```python
from build123d import *

# Parameters (mm, degrees)
SKETCH_2_R      = 3
EXTRUDE_1_DEPTH = 1.6


with BuildPart() as part:
    # 스케치2 → 보스-돌출1 (new body)
    with BuildSketch(Plane(origin=(0, 0, 0), x_dir=(0, 0, -1), z_dir=(1, 0, 0))):
        with BuildLine():
            Line((-13.45, 1.3), (-11.65, 1.3))
            Line((-11.65, 1.3), (-11.65, 0.5))
            Line((-11.65, 0.5), (-7.05, 0.5))
            Line((-7.05, 0.5), (-7.05, 1.3))
            Line((-7.05, 1.3), (-2, 1.3))
            Line((-2, 1.3), (-2, 2.063932023))
            ThreePointArc((-2, 2.063932023), (0, 7.3), (2, 2.063932023))
            Line((2, 2.063932023), (2, 1.3))
            Line((2, 1.3), (7.05, 1.3))
            Line((7.05, 1.3), (7.05, 0.5))
            Line((7.05, 0.5), (11.65, 0.5))
            Line((11.65, 0.5), (11.65, 1.3))
            Line((11.65, 1.3), (13.45, 1.3))
            Line((13.45, 1.3), (13.45, 10.3))
            Line((13.45, 10.3), (-11.45, 10.3))
            Line((-11.45, 10.3), (-11.45, 12.3))
            Line((-11.45, 12.3), (-13.45, 12.3))
            Line((-13.45, 12.3), (-13.45, 1.3))
        make_face()
        with Locations((-7.05, 6.25)):
            Circle(SKETCH_2_R, mode=Mode.SUBTRACT)
        with Locations((7.05, 6.25)):
            Circle(SKETCH_2_R, mode=Mode.SUBTRACT)
    extrude(amount=EXTRUDE_1_DEPTH)


solid = part.part
```
Geometry: final body of the model. Coordinates: model frame, mm. A direction names the side the tool comes from. Coordinates: 2 decimals unless noted, no trailing zeros. Order: outer loops, then holes, each group sorted by start corner. A loop starts at its lowest first (then second) coordinate and runs counter-clockwise, first axis right, second up. Notation, with made-up numbers: (-38, 30) - (15, 30) arc R37 ccw to (15, 66) - close; hole circle Ø4 at (38.25, 59). An arc over 180 degrees is marked (long way). Return JSON: item names as keys, results as strings. Group by question number.
1. Set-up query: faces 4 (the face through (1, 0.5, -9)), 5 (the face through (1, 1.3, -4)), 6 (the face through (1, 10.3, -1)), 7 (the face through (1, 1.3, -13)), 8 (the face through (1, 1.3, 13)). Return all of +Z, -Z, +X, -X, +Y, -Y with unobstructed straight access to the full face (end or side cutting, diameter ignored); none if empty.
2. Cut plane B-B (x = 0.85). Output: boundary loops of the cut face in (y, z).
3. Cut plane D-D (z = 9). Output: boundary loops of the cut face in (x, y), plus the area to 3 significant figures.
4. Material intervals for line 1 along Z through (x, y) = (0.6, 4); line 2 along Z through (x, y) = (0.25, 4.25); line 3 along Z through (x, y) = (0.45, 9), sorted ascending. Write a range as [from, to].
5. Pull-direction query (Z, two-part tool) for faces 1 (the face through (1, 1.3, 5)), 2 (the face through (1, 7, 13.45)), 3 (the face through (1, 11, 11.45)); classes: pulls with the +Z half, pulls with the -Z half, needs draft (parallel to the pull), parting line crosses it, or undercut.
6. Cut plane A-A (y = 2.5). Output: boundary loops of the cut face in (x, z), plus the area to 3 significant figures.
7. Cut plane C-C (y = 6.25). Output: boundary loops of the cut face in (x, z), plus the area to 3 significant figures.
8. Pin query (flat end, axial travel): pin 1 (0.8 mm diameter, centred on x = 0.5, z = 12.5, fed in from -Y). Return the tip coordinate at first contact, or that it passes through.
Resolved:
{
 "1": {"face 4": "+Z, -Z, +X, -X, -Y", "face 5": "+X, -X, -Y", "face 6": "-Z, +X, -X, +Y", "face 7": "-Z, +X, -X, -Y", "face 8": "+Z, +X, -X, -Y"},
 "2": {"outline": "(0.5, -11.65) - (1.3, -11.65) - (1.3, -13.45) - (10.3, -13.45) - (10.3, 11.45) - (12.3, 11.45) - (12.3, 13.45) - (1.3, 13.45) - (1.3, 11.65) - (0.5, 11.65) - (0.5, 7.05) - (1.3, 7.05) - (1.3, 2) - (2.06, 2) arc R3 cw (long way) to (2.06, -2) - (1.3, -2) - (1.3, -7.05) - (0.5, -7.05) - close; hole circle Ø6 at (6.25, -7.05); hole circle Ø6 at (6.25, 7.05)"},
 "3": {"outline": "(0, 0.5) - (1.6, 0.5) - (1.6, 3.97) - (0, 3.97) - close; (0, 8.53) - (1.6, 8.53) - (1.6, 10.3) - (0, 10.3) - close", "area": "8.38 mm²"},
 "4": {"line 1": "z = [-13.45, -9.03], [-5.07, -2.98], [2.98, 5.07], [9.03, 13.45]", "line 2": "z = [-13.45, -9.29], [-4.81, -3], [3, 4.81], [9.29, 13.45]", "line 3": "z = [-13.45, -8.25], [-5.85, 5.85], [8.25, 13.45]"},
 "5": {"face 1": "undercut", "face 2": "pulls with the +Z half", "face 3": "pulls with the -Z half"},
 "6": {"outline": "(0, -13.45) - (1.6, -13.45) - (1.6, -2.4) - (0, -2.4) - close; (0, 2.4) - (1.6, 2.4) - (1.6, 13.45) - (0, 13.45) - close", "area": "35.4 mm²"},
 "7": {"outline": "(0, -13.45) - (1.6, -13.45) - (1.6, -10.05) - (0, -10.05) - close; (0, -4.05) - (1.6, -4.05) - (1.6, -2.28) - (0, -2.28) - close; (0, 2.28) - (1.6, 2.28) - (1.6, 4.05) - (0, 4.05) - close; (0, 10.05) - (1.6, 10.05) - (1.6, 13.45) - (0, 13.45) - close", "area": "16.5 mm²"},
 "8": {"pin 1": "stops at y = 1.3"}
}
